Can you work these out from the model? Positions are in its coordinate system, mm. A direction names the side the tool comes from. Round coordinates to 2 decimals unless told otherwise and drop trailing zeros. Loops run counter-clockwise (first coordinate to the right, second up) from the corner with the lowest first, then second, coordinate; pieces in that order, holes last. Notation, with made-up numbers: M 77.25,37 L 122.25,37 A19 cw 122.25,55 Z; hole C 87.25,19 d8. An arc over 180 degrees is marked long. Use a Markdown table: item, result. Add a question column.
```python
from build123d import *

# Parameters (mm, degrees)
SKETCH1_R           = 19.05
SKETCH1_R_2         = 5.08
BOSS_EXTRUDE2_DEPTH = 10.16
CUT_EXTRUDE2_DEPTH  = 10.16


with BuildPart() as part:
    # Sketch1 → Boss-Extrude2 (new body)
    with BuildSketch(Plane.XY):
        with Locations((-23.004204789, 15.609996107)):
            Circle(SKETCH1_R)
        with Locations((-23.004204789, 15.609996107)):
            Circle(SKETCH1_R_2, mode=Mode.SUBTRACT)
    extrude(amount=BOSS_EXTRUDE2_DEPTH)

    # Sketch3 → Cut-Extrude2 (cut)
    with BuildSketch(Plane.XY.offset(10.16)):
        Polygon((-23.004204789, 23.186689095), (-28.334456331, 29.08814957), (-23.004204789, 29.08814957), align=None)
        Polygon((-12.466560086, 24.013487339), (-17.080507678, 20.333986917), (-15.789917564, 28.180845804), align=None)
        Polygon((-9.863976773, 12.61082481), (-15.617475313, 13.924023307), (-8.677884222, 17.807435817), align=None)
        Polygon((-17.156253168, 3.46659944), (-19.716800906, 8.783631603), (-12.353862471, 5.779308909), align=None)
        Polygon((-28.85215641, 3.46659944), (-26.291608673, 8.783631603), (-24.049765713, 1.153889971), align=None)
        Polygon((-36.144432805, 12.61082481), (-30.390934265, 13.924023307), (-34.958340254, 7.414213804), align=None)
        Polygon((-33.541849492, 24.013487339), (-28.9279019, 20.333986917), (-36.86520697, 19.846128875), align=None)
    extrude(amount=-CUT_EXTRUDE2_DEPTH, mode=Mode.SUBTRACT)


solid = part.part
```
(1) Suppose I cut it at A-A on z = 4. Count the separate pieces of the cut face and the enclosed holes in it, and give its area (3 significant figures).
(2) I'm going to push flat-ended pins straight in: pin 1 (6 mm diameter, centred on x = -8, z = 4, fed in from -Y); pin 2 (4 mm diameter, centred on x = -27.5, y = 6, fed in from -Z); pin 3 (1.6 mm diameter, centred on x = -25.5, z = 4.5, fed in from -Y); pin 4 (3 mm diameter, centred on y = 24.5, z = 7.5, fed in from -X). Where does each tip first touch, or does it pass through?
(3) On a 3-axis mill with a long thin cutter (end or side, diameter ignored), from which of +Z, -Z, +X, -X, +Y, -Y can I reach the whole of each face in a straight line? I mean faces 1 (the face through (-19, 12, 0)), 2 (the face through (-26.417, 2.294, 5.151)). Say none if no direction works.
(4) If I drill on probe 1 along Y at (x, z) = (-15, 7) (3 decimals); probe 2 along X at (y, z) = (17, 2); probe 3 along X at (y, z) = (12.5, 2.75), over which ranges is the centre line in solid material (lowest first)? Write a range as [from, to].
(5) Suppose I cut it at D-D on y = 32. List the corners of the cut face in (x, z) for me, and give its area (3 significant figures).
(6) Suppose I cut it at C-C on y = 25. List the corners of the cut face in (x, z) for me, and give its area (3 significant figures).
(7) Suppose I cut it at B-B on x = -31. List the corners of the cut face in (y, z) for me (3 decimals).
(8) Thinking about a two-plate mould opening in Y: for faces 3 (the face through (-25.48, 34.5, 5.01)), 4 (the face through (-31.27, 22.2, 5.15)), 5 (the face through (-19, 12, 10.16)), 6 (the face through (-16.444, 24.202, 5.151)), which applies, released by +Y, released by -Y, zero draft, split by the parting line, or undercut?
Results below:
| question | item | result |
|---|---|---|
| 1 | separate pieces | 1 |
| 1 | enclosed holes | 8 |
| 1 | area | 949 mm² |
| 2 | pin 1 | stops at y = 0.82 |
| 2 | pin 2 | stops at z = 0 |
| 2 | pin 3 | stops at y = -3.36 |
| 2 | pin 4 | stops at x = -40.56 |
| 3 | face 1 | -Z, +X, -X, +Y, -Y |
| 3 | face 2 | +Z, -Z |
| 4 | probe 1 | y = [-1.677, 4.505], [6.859, 13.783], [14.27, 21.993], [27.19, 32.897] |
| 4 | probe 2 | x = [-42, -27.89], [-18.12, -10.12], [-8.86, -4] |
| 4 | probe 3 | x = [-41.8, -36.12], [-31.39, -27.02], [-18.99, -4.21] |
| 5 | outline | M -32.71,0 L -13.29,0 L -13.29,10.16 L -32.71,10.16 Z |
| 5 | area | 197 mm² |
| 6 | outline | M -39.58,0 L -24.64,0 L -24.64,10.16 L -39.58,10.16 Z; M -23,0 L -16.31,0 L -16.31,10.16 L -23,10.16 Z; M -13.25,0 L -6.43,0 L -6.43,10.16 L -13.25,10.16 Z |
| 6 | area | 289 mm² |
| 7 | outline | M -1.681,0 L 13.056,0 L 13.056,10.16 L -1.681,10.16 Z; M 13.785,0 L 20.207,0 L 20.207,10.16 L 13.785,10.16 Z; M 21.986,0 L 32.901,0 L 32.901,10.16 L 21.986,10.16 Z |
| 8 | face 3 | split by the parting line |
| 8 | face 4 | undercut |
| 8 | face 5 | zero draft |
| 8 | face 6 | undercut |
